CAD build for the part. Positions are in the model's coordinates, mm. A direction names the side the tool comes from. Give positions to 0.01 mm unless a question says otherwise; leave off trailing zeros. Loops run counter-clockwise (first coordinate to the right, second up) from the corner with the lowest first, then second, coordinate; pieces in that order, holes last. Notation, with made-up numbers: (16, -10) -> (59, -10) arc R8 cw to (59, 1) -> close; hole circle Ø10 at (-27, 48). An arc over 180 degrees is marked (long way). Use one line per item in the form item = value.
```python
from build123d import *

# Parameters (mm, degrees)
BOSS_EXTRU_1_DEPTH      = 40
ESQUISSE2_R             = 1.75
ENL_V_MAT_EXTRU_1_DEPTH = 92.923881554
ESQUISSE5_R             = 6.3126
ENL_V_MAT_EXTRU_2_DEPTH = 162.632298752


with BuildPart() as part:
    # Esquisse1 → Boss.-Extru.1 (new body)
    with BuildSketch(Plane.XY):
        Polygon((-65, 45), (-75, 45), (-75, 0), (75, 0), (75, 45), (65, 45), (65, 10), (-65, 10), align=None)
    extrude(amount=BOSS_EXTRU_1_DEPTH)

    # Esquisse2 → Enlèv. mat.-Extru.1 (cut, through all)
    with BuildSketch(Plane(origin=(0, 10, 0), x_dir=(1, 0, 0), z_dir=(0, 1, 0))):
        with Locations(Location((-13.788582233, -6.211417767, 0), (0, 0, 270))):
            Circle(ESQUISSE2_R)
        with Locations(Location((13.788582233, -6.211417767, 0), (0, 0, 270))):
            Circle(ESQUISSE2_R)
        with Locations(Location((13.788582233, -33.788582233, 0), (0, 0, 270))):
            Circle(ESQUISSE2_R)
        with Locations(Location((-13.788582233, -33.788582233, 0), (0, 0, 270))):
            Circle(ESQUISSE2_R)
    extrude(amount=-ENL_V_MAT_EXTRU_1_DEPTH, mode=Mode.SUBTRACT)

    # Esquisse5 → Enlèv. mat.-Extru.2 (cut, through all)
    with BuildSketch(Plane.ZY.offset(75)):
        with Locations((20, 33.0538058)):
            Circle(ESQUISSE5_R)
    extrude(amount=-ENL_V_MAT_EXTRU_2_DEPTH, mode=Mode.SUBTRACT)


solid = part.part
```
1. Drop a flat-ended pin along its axis: P1, Ø4, axis at x = -13.79, z = 33.79, coming from the +Y side. Give the stop position or say it passes through.
Result sheet:
P1 = 10
2. Drill centre lines: line 1 (Z direction, x = 13.5, y = 7); line 2 (X direction, y = 42, z = 33); line 3 (Y direction, x = -31, z = 11). Where is each one in solid material? Low to high.
Result sheet:
line_1 = 0 to 4.49, 7.94 to 32.06, 35.51 to 40
line_2 = -75 to -65, 65 to 75
line_3 = 0 to 10
3. Cut at C-C, the plane x = -57. Write the cut outline in (y, z).
Result sheet:
outline = (0, 0) -> (10, 0) -> (10, 40) -> (0, 40) -> close
4. Cut at D-D, the plane z = 33.5. Write the cut outline in (x, y).
Result sheet:
outline = (-75, 0) -> (-15.51, 0) -> (-15.51, 10) -> (-65, 10) -> (-65, 45) -> (-75, 45) -> close; (-12.06, 0) -> (12.06, 0) -> (12.06, 10) -> (-12.06, 10) -> close; (15.51, 0) -> (75, 0) -> (75, 45) -> (65, 45) -> (65, 10) -> (15.51, 10) -> close
5. Cut at B-B, the plane z = 20. Write the cut outline in (x, y).
Result sheet:
outline = (-75, 0) -> (75, 0) -> (75, 26.74) -> (65, 26.74) -> (65, 10) -> (-65, 10) -> (-65, 26.74) -> (-75, 26.74) -> close; (-75, 39.37) -> (-65, 39.37) -> (-65, 45) -> (-75, 45) -> close; (65, 39.37) -> (75, 39.37) -> (75, 45) -> (65, 45) -> close
6. Mould opens along Y. For faces 1 (the flat face through (-70, 45, 20)), 2 (the flat face through (-65, 23, 20)), 3 (the cylindrical face through (-70.07, 38.38, 23.39)) say: pulls with the +Y half, pulls with the -Y half, needs draft (parallel to the pull), parting line crosses it, or undercut.
Result sheet:
face_1 = pulls with the +Y half
face_2 = needs draft
face_3 = undercut
7. Cut at A-A, the plane y = 18.5. Write the cut outline in (x, z).
Result sheet:
outline = (-75, 0) -> (-65, 0) -> (-65, 40) -> (-75, 40) -> close; (65, 0) -> (75, 0) -> (75, 40) -> (65, 40) -> close
8. Tool access for faces 4 (the flat face through (1, 10, 20)), 5 (the cylindrical face through (69.93, 38.38, 23.39)): list every direction of +Z, -Z, +X, -X, +Y, -Y with a clear straight run to the whole face (end or side of a thin tool).
Result sheet:
face_4 = +Z, -Z, +Y
face_5 = +X, -X
